```python
from build123d import *

# Parameters (mm, degrees)
EXTRUDE_1_DEPTH     = 4
SKETCH_2_R          = 10
SKETCH_2_R_2        = 5
EXTRUDE_2_DEPTH     = 10
SKETCH_3_R          = 1.8
CUT_EXTRUDE_1_DEPTH = 13


with BuildPart() as part:
    # 草图1 → 凸台-拉伸1 (new body)
    with BuildSketch(Plane.XY):
        with BuildLine():
            ThreePointArc((-20.5, 0), (0, -20.5), (20.5, 0))
            ThreePointArc((20.5, 0), (0, 20.5), (-20.5, 0))
        make_face()
        with BuildLine():
            ThreePointArc((-16.5, 0), (-15, -1.5), (-13.5, 0))
            ThreePointArc((-13.5, 0), (-15, 1.5), (-16.5, 0))
        make_face(mode=Mode.SUBTRACT)
        with BuildLine():
            ThreePointArc((-1.5, -15), (0, -16.5), (1.5, -15))
            ThreePointArc((1.5, -15), (0, -13.5), (-1.5, -15))
        make_face(mode=Mode.SUBTRACT)
        with BuildLine():
            ThreePointArc((13.5, 0), (15, -1.5), (16.5, 0))
            ThreePointArc((16.5, 0), (15, 1.5), (13.5, 0))
        make_face(mode=Mode.SUBTRACT)
        with BuildLine():
            ThreePointArc((-1.5, 15), (0, 13.5), (1.5, 15))
            ThreePointArc((1.5, 15), (0, 16.5), (-1.5, 15))
        make_face(mode=Mode.SUBTRACT)
        with BuildLine():
            ThreePointArc((-5, 0), (0, -5), (5, 0))
            ThreePointArc((5, 0), (0, 5), (-5, 0))
        make_face(mode=Mode.SUBTRACT)
    extrude(amount=EXTRUDE_1_DEPTH)

    # 草图2 → 凸台-拉伸2 (add)
    with BuildSketch(Plane.XY.offset(4)):
        Circle(SKETCH_2_R)
        Circle(SKETCH_2_R_2, mode=Mode.SUBTRACT)
    extrude(amount=EXTRUDE_2_DEPTH)

    # 草图3 → 切除-拉伸1 (cut)
    with BuildSketch(Plane(origin=(0, 0, 0), x_dir=(1, 0, 0), z_dir=(0, 1, 0))):
        with Locations(Location((0, -9, 0), (0, 0, 270))):
            Circle(SKETCH_3_R)
    extrude(amount=-CUT_EXTRUDE_1_DEPTH, mode=Mode.SUBTRACT)


solid = part.part
```
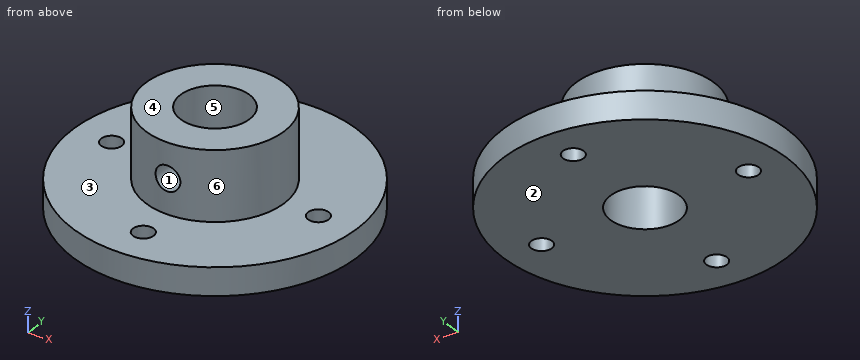
CAD build for the part. Positions are in the model's coordinates, mm. Face numbers are marked on the shaded views. A direction names the side the tool comes from. Coordinates: 2 decimals unless noted, no trailing zeros. Loops run counter-clockwise (first coordinate to the right, second up) from the corner with the lowest first, then second, coordinate; pieces in that order, holes last. Notation, with made-up numbers: (21, -36) - (79, -36) arc R16 ccw to (79, -23) - close; hole circle Ø1 at (85.25, 36.5). An arc over 180 degrees is marked (long way). Use CSV: the item, a comma, the result in double quotes. Start each with the question number.
Q1. Two-plate mould, pull along X, no slides. Class the marked faces 4, 5 and 6: +X half, -X half, draft (parallel to the pull), parting line (faces both ways), or undercut.
Q2. Cut at A-A, the plane x = 0. List the corners of the cut face in (y, z), then the cut area to 3 significant figures.
Q3. Drop flat-ended pins along their axis: P1, Ø3, axis at x = 0, z = 9, coming from the -Y side; P2, Ø8, axis at y = -2.5, z = 2, coming from the -X side; P3, Ø4, axis at y = 10, z = 8.5, coming from the +X side; P4, Ø1, axis at y = -8, z = 5.5, coming from the -X side. Give the stop position or say it passes through.
Q4. Probe probe 1 along Y at (x, z) = (0, 2.25); probe 2 along Z at (x, y) = (0, -8); probe 3 along Y at (x, z) = (0, 6.25). List the from-to ranges inside material, lowest first. Write a range as from..to.
Q5. Cut at C-C, the plane x = -14. List the corners of the cut face in (y, z).
Q6. Cut at D-D, the plane x = 8. List the corners of the cut face in (y, z).
Q7. Cut at B-B, the plane y = 15. List the corners of the cut face in (x, z).
Q8. 3-axis set-ups, long thin cutter, end or side, ignore diameter. For the marked faces 1, 2 and 3: which of +Z, -Z, +X, -X, +Y, -Y reach the whole face in a straight line?
Here are the results:
1,face 4,"draft"
1,face 5,"undercut"
1,face 6,"parting line"
2,outline,"(-20.5, 0) - (-16.5, 0) - (-16.5, 4) - (-20.5, 4) - close; (-13.5, 0) - (-5, 0) - (-5, 7.2) - (-10, 7.2) - (-10, 4) - (-13.5, 4) - close; (-10, 10.8) - (-5, 10.8) - (-5, 14) - (-10, 14) - close; (5, 0) - (13.5, 0) - (13.5, 4) - (10, 4) - (10, 14) - (5, 14) - close; (16.5, 0) - (20.5, 0) - (20.5, 4) - (16.5, 4) - close"
2,area,"182 mm2"
3,P1,"y = 4.77"
3,P2,"x = -20.5"
3,P3,"x = 6"
3,P4,"x = -6.61"
4,probe 1,"-20.5..-16.5, -13.5..-5, 5..13.5, 16.5..20.5"
4,probe 2,"0..7.2, 10.8..14"
4,probe 3,"-10..-5, 5..10"
5,outline,"(-14.97, 0) - (-1.12, 0) - (-1.12, 4) - (-14.97, 4) - close; (1.12, 0) - (14.97, 0) - (14.97, 4) - (1.12, 4) - close"
6,outline,"(-18.87, 0) - (18.87, 0) - (18.87, 4) - (6, 4) - (6, 14) - (-6, 14) - (-6, 4) - (-18.87, 4) - close"
7,outline,"(-13.97, 0) - (-1.5, 0) - (-1.5, 4) - (-13.97, 4) - close; (1.5, 0) - (13.97, 0) - (13.97, 4) - (1.5, 4) - close"
8,face 1,"-Y"
8,face 2,"-Z, +X, -X, +Y, -Y"
8,face 3,"+Z"
